Check sheet for the modelled part. Datum: model origin and axes. Units: mm. Face numbers are marked on the shaded views. A direction names the side the tool comes from. Round coordinates to 2 decimals unless told otherwise and drop trailing zeros. Loops run counter-clockwise (first coordinate to the right, second up) from the corner with the lowest first, then second, coordinate; pieces in that order, holes last. Notation, with made-up numbers: (83, 40.5) - (108, 40.5) arc R9 cw to (108, 51.5) - close; hole circle Ø2 at (0, 56). An arc over 180 degrees is marked (long way). Put each result on its own line as item: value.
```python
from build123d import *

# Parameters (mm, degrees)
RESSALTO_EXTRUS_O2_DEPTH = 27
ESBO_O2_R                = 4.6
CORTE_EXTRUS_O1_DEPTH    = 35
CORTE_EXTRUS_O3_DEPTH    = 60
ESBO_O7_W                = 27
ESBO_O7_H                = 35
RESSALTO_EXTRUS_O3_DEPTH = 5
ESBO_O8_R                = 3
CORTE_EXTRUS_O4_DEPTH    = 123.96442575
FILETE1_R                = 30
ESBO_O12_R               = 3.5
CORTE_EXTRUS_O5_DEPTH    = 113.730874209


with BuildPart() as part:
    # Esboço1 → Ressalto-extrusão2 (new body)
    with BuildSketch(Plane.XY):
        with BuildLine():
            Line((-85, -14), (85, -14))
            Line((85, -14), (85, -10.332291626))
            ThreePointArc((85, -10.332291626), (79.690886502, 21.313445506), (48.447441117, 14))
            Line((48.447441117, 14), (-85, 14))
            Line((-85, 14), (-85, -14))
        make_face()
    extrude(amount=RESSALTO_EXTRUS_O2_DEPTH)

    # Esboço2 → Corte-extrusão1 (cut)
    with BuildSketch(Plane.XY.offset(27)):
        with Locations((67.5, 3)):
            Circle(ESBO_O2_R)
    extrude(amount=-CORTE_EXTRUS_O1_DEPTH, mode=Mode.SUBTRACT)

    # Esboço6 → Corte-extrusão3 (cut)
    with BuildSketch(Plane.ZY.offset(85)):
        Polygon((5, -9), (22, -9), (27, -9), (27, 14), (0, 14), (0, -9), align=None)
    extrude(amount=-CORTE_EXTRUS_O3_DEPTH, mode=Mode.SUBTRACT)

    # Esboço7 → Ressalto-extrusão3 (add)
    with BuildSketch(Plane.ZY.offset(25)):
        with Locations((13.5, 31.5)):
            Rectangle(ESBO_O7_W, ESBO_O7_H)
    extrude(amount=-RESSALTO_EXTRUS_O3_DEPTH)

    # Esboço8 → Corte-extrusão4 (cut, through all)
    with BuildSketch(Plane(origin=(-20, 0, 0), x_dir=(0, 0, -1), z_dir=(1, 0, 0))):
        with Locations((-6.646583991, 43.091925341)):
            Circle(ESBO_O8_R)
        with Locations(Location((-6.646583991, 30.908074659, 0), (0, 0, 180))):
            Circle(ESBO_O8_R)
    extrude(amount=-CORTE_EXTRUS_O4_DEPTH, mode=Mode.SUBTRACT)

    # Filete1
    # the kernel refuses this fillet: 30 mm, written as the material it takes off along each edge
    with BuildSketch(Plane(origin=(-85, -14, -41.457809879), x_dir=(0, 1, 0), z_dir=(0, 0, 1))) as filete1_piece_1:
        with BuildLine():
            CenterArc((30, -16.583123952), FILETE1_R, 146.442690238, 33.557309762)
            Line((0, -16.583123952), (-0.6, -16.583123952))
            Line((-0.6, -16.583123952), (-0.6, 0))
            Line((-0.6, 0), (0, 0.6))
            ThreePointArc((0, 0.6), (2.5, 0.6), (4.5, 0.331662479))
            Line((4.5, 0.331662479), (5, 0))
        make_face()
    extrude(amount=109.915619759, mode=Mode.SUBTRACT)

    # Esboço12 → Corte-extrusão5 (cut, through all)
    with BuildSketch(Plane.XZ.offset(14)):
        with Locations((88.855428665, 13.5)):
            Circle(ESBO_O12_R)
    extrude(amount=-CORTE_EXTRUS_O5_DEPTH, mode=Mode.SUBTRACT)


solid = part.part
```
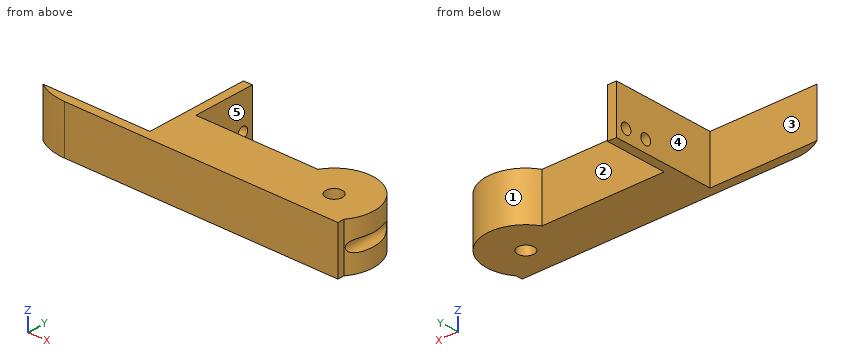
Item 1: Go/stop test with flat-tipped pins: pin 1 (8 mm diameter, centred on y = 25.5, z = 15, fed in from -X); pin 2 (8.5 mm diameter, centred on x = 67.5, y = 3, fed in from +Z); pin 3 (8 mm diameter, centred on x = -64.5, z = 16, fed in from +Y); pin 4 (13.5 mm diameter, centred on y = 33.5, z = 19.5, fed in from +X). Record where each tip stops, or that it passes through.
Filled sheet:
pin 1: x = -25
pin 2: through
pin 3: y = -9
pin 4: x = -20
Item 2: Section check C-C on y = 3. Enter the section's corners in (x, z).
Filled sheet:
outline: (-25, 0) - (62.9, 0) - (62.9, 27) - (-25, 27) - close; (72.1, 0) - (89.5, 0) - (89.5, 10.06) arc R3.5 cw (long way) to (89.5, 16.94) - (89.5, 27) - (72.1, 27) - close
Item 3: Section check A-A on z = 13.5. Enter the section's corners in (x, y).
Filled sheet:
outline: (-85, -9) arc R30 ccw to (-68.42, -14) - (85, -14) - (85, -10.33) arc R22 ccw to (85.36, -9.85) - (85.36, 15.85) arc R22 ccw to (48.45, 14) - (-20, 14) - (-20, 49) - (-25, 49) - (-25, -9) - close; hole circle Ø9.2 at (67.5, 3)
Item 4: Section check B-B on x = 67.5. Enter the section's corners in (y, z).
Filled sheet:
outline: (-14, 0) - (-1.6, 0) - (-1.6, 27) - (-14, 27) - close; (7.6, 0) - (25, 0) - (25, 27) - (7.6, 27) - close
Item 5: Release check for a two-part mould opening along X. For the marked faces 3, 4 and 5 record: +X half, -X half, draft (parallel to the pull), parting line (faces both ways), or undercut.
Filled sheet:
face 3: draft
face 4: -X half
face 5: undercut
Item 6: Thickness scan on line 1 (Y direction, x = 35, z = 20.5); line 2 (Y direction, x = -30, z = 22); line 3 (X direction, y = 19, z = 11.5). Record the ranges inside material, lowest first. Write a range as from..to.
Filled sheet:
line 1: -14..14
line 2: -14..-9
line 3: -25..-20, 52.4..82.6
Item 7: Tool access check on the marked faces 1 and 2. Record the directions out of +Z, -Z, +X, -X, +Y, -Y that give a thin tool (end or side, any length) a straight path to the whole face; none if there is none.
Filled sheet:
face 1: +Z, -Z
face 2: +Z, -Z, +Y
Item 8: Section check D-D on z = 21.25. Enter the section's corners in (x, y), then the cut area to 3 significant figures.
Filled sheet:
outline: (-85, -9) arc R30 ccw to (-68.42, -14) - (85, -14) - (85, -10.33) arc R22 ccw (long way) to (48.45, 14) - (-20, 14) - (-20, 49) - (-25, 49) - (-25, -9) - close; hole circle Ø9.2 at (67.5, 3)
area: 3,840 mm²
